from build123d import *

# Parameters (mm, degrees)
SKETCH1_W           = 20
SKETCH1_H           = 20
BOSS_EXTRUDE1_DEPTH = 1
SKETCH2_W           = 20
SKETCH2_H           = 20
SKETCH2_R           = 2.5
BOSS_EXTRUDE2_DEPTH = 1
BOSS_EXTRUDE3_DEPTH = 20
BOSS_EXTRUDE4_START = -19
BOSS_EXTRUDE4_DEPTH = 1
BOSS_EXTRUDE5_DEPTH = 20


with BuildPart() as part:
    # Sketch1 → Boss-Extrude1 (new body)
    with BuildSketch(Plane(origin=(0, 0, 0), x_dir=(1, 0, 0), z_dir=(0, 1, 0))):
        Rectangle(SKETCH1_W, SKETCH1_H)
    extrude(amount=BOSS_EXTRUDE1_DEPTH)

    # Sketch2 → Boss-Extrude2 (add)
    with BuildSketch(Plane.XY.offset(10)):
        with Locations((0, 10)):
            Rectangle(SKETCH2_W, SKETCH2_H)
        with Locations((0, 10)):
            Circle(SKETCH2_R, mode=Mode.SUBTRACT)
    extrude(amount=-BOSS_EXTRUDE2_DEPTH)

    # Sketch3 → Boss-Extrude3 (add)
    with BuildSketch(Plane(origin=(10, 0, 0), x_dir=(0, 0, -1), z_dir=(1, 0, 0))):
        Polygon((-9, 4), (-6, 1), (-9, 1), align=None)
    extrude(amount=-BOSS_EXTRUDE3_DEPTH)

    # Sketch3<2> → Boss-Extrude4 (add)
    with BuildSketch(Plane(origin=(10, 0, 0), x_dir=(0, 0, -1), z_dir=(1, 0, 0)).offset(BOSS_EXTRUDE4_START)):
        Polygon((-9, 4), (-6, 1), (-9, 1), align=None)
    extrude(amount=-BOSS_EXTRUDE4_DEPTH)

    # Sketch4 → Boss-Extrude5 (add)
    with BuildSketch(Plane(origin=(10, 0, 0), x_dir=(0, 0, -1), z_dir=(1, 0, 0))):
        Polygon((-2, 0), (-2, -2), (-4.5, -2), (-4.5, -3.436102186), (4.5, -3.436102186), (4.5, -2), (2, -2), (2, 0), align=None)
    extrude(amount=-BOSS_EXTRUDE5_DEPTH)


solid = part.part
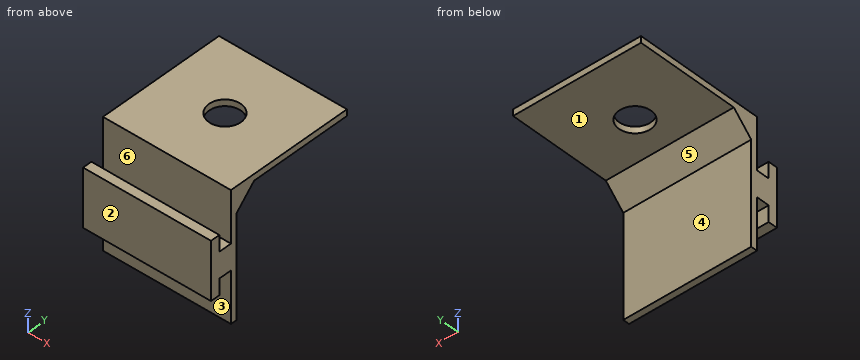
Model file for the job. Use its own axes, mm. Face numbers are marked on the shaded views. A direction names the side the tool comes from. Round coordinates to 2 decimals unless told otherwise and drop trailing zeros. Order: outer loops, then holes, each group sorted by start corner. A loop starts at its lowest first (then second) coordinate and runs counter-clockwise, first axis right, second up.
(1) Drill centre lines: line 1 (Y direction, x = 3, z = -3); line 2 (Y direction, x = 0, z = 9.4); line 3 (Z direction, x = 4, y = 5). Where is each one in solid material? Low to high.
(2) Band-saw the part on B-B (y = 10). List the corners of the cut face in (x, z).
(3) 3-axis set-ups, long thin cutter, end or side, ignore diameter. For the marked faces 5 and 6: which of +Z, -Z, +X, -X, +Y, -Y reach the whole face in a straight line?
(4) Band-saw the part on A-A (z = 2.5). List the corners of the cut face in (x, y).
(5) Pin check, flat tips, straight feed: pin 1 (1 mm diameter, centred on x = -2.5, y = 12.5, fed in from -Z); pin 2 (1 mm diameter, centred on x = 5, y = -1, fed in from -Z); pin 3 (10 mm diameter, centred on y = 15, z = 8, fed in from -X); pin 4 (3 mm diameter, centred on x = 0, z = 3.5, fed in from +Y). Stop position of each tip, or through.
(6) Band-saw the part on D-D (x = -3.25). List the corners of the cut face in (y, z), then the cut area to 3 significant figures.
(7) Band-saw the part on C-C (x = 0). List the corners of the cut face in (y, z).
(8) Pull direction Y, two halves, no side cores. Call the marked faces 1, 2, 3 and 4: released by +Y, released by -Y, zero draft, split by the parting line, or undercut.
Verdict:
1. line 1: y = -3.44 to -2, 0 to 1
1. line 2: y = 0 to 7.5, 12.5 to 20
1. line 3: z = 9 to 10
2. outline: (-10, 9) - (-2.5, 9) - (-2.5, 10) - (-10, 10) - close; (2.5, 9) - (10, 9) - (10, 10) - (2.5, 10) - close
3. face 5: -Z, +X, -X, +Y
3. face 6: +Z, +X, -X
4. outline: (-10, -3.44) - (10, -3.44) - (10, -2) - (-10, -2) - close; (-10, 0) - (10, 0) - (10, 1) - (-10, 1) - close
5. pin 1: stops at z = 9
5. pin 2: stops at z = -2
5. pin 3: stops at x = -10
5. pin 4: stops at y = 1
6. outline: (-3.44, -4.5) - (-2, -4.5) - (-2, -2) - (0, -2) - (0, -10) - (1, -10) - (1, 6) - (4, 9) - (20, 9) - (20, 10) - (0, 10) - (0, 2) - (-2, 2) - (-2, 4.5) - (-3.44, 4.5) - close
6. area: 64.4 mm2
7. outline: (-3.44, -4.5) - (-2, -4.5) - (-2, -2) - (0, -2) - (0, -10) - (1, -10) - (1, 6) - (4, 9) - (7.5, 9) - (7.5, 10) - (0, 10) - (0, 2) - (-2, 2) - (-2, 4.5) - (-3.44, 4.5) - close; (12.5, 9) - (20, 9) - (20, 10) - (12.5, 10) - close
8. face 1: zero draft
8. face 2: released by -Y
8. face 3: undercut
8. face 4: released by +Y
